Can you work these out from the model? Positions are in its coordinate system, mm. Face numbers are marked on the shaded views. A direction names the side the tool comes from. Round coordinates to 2 decimals unless told otherwise and drop trailing zeros. Order: outer loops, then holes, each group sorted by start corner. A loop starts at its lowest first (then second) coordinate and runs counter-clockwise, first axis right, second up. Notation, with made-up numbers: (14.5, 41.25) -> (44.5, 41.25) arc R25 cw to (44.5, 56.25) -> close; hole circle Ø6 at (55.25, 16). An arc over 180 degrees is marked (long way). Use a Markdown table: item, result. Add a question column.
Q1. If we section it at D-D on y = 15: List the corners of the cut face in (x, z) for me.
Q2. If we section it at A-A on z = -19.5: List the corners of the cut face in (x, y) for me.
Q3. For the marked faces 1, 2, 3, 4 and 5, which set-ups out of +Z, -Z, +X, -X, +Y, -Y let a thin tool reach every point of the face, with its end or its side?
Q4. I need wall thicknesses on line 1 along X through (y, z) = (-17, -2); line 2 along Z through (x, y) = (-14.5, -19). Which ranges of each line are inside material? Lowest first, please. Write a range as [from, to].
Q5. I'm going to push flat-ended pins straight in: pin 1 Ø1.5 at (x, y) = (-5, -7) entering from +Z; pin 2 Ø6 at (y, z) = (5, 5.5) entering from +X; pin 3 Ø6 at (y, z) = (-6, -14.5) entering from -X. Where does each tip first touch, or does it pass through?
Q6. We'd pull the mould along X, two halves only. Please class the marked faces 6, 7, 8 and 9: +X half, -X half, draft (parallel to the pull), parting line (faces both ways), or undercut.
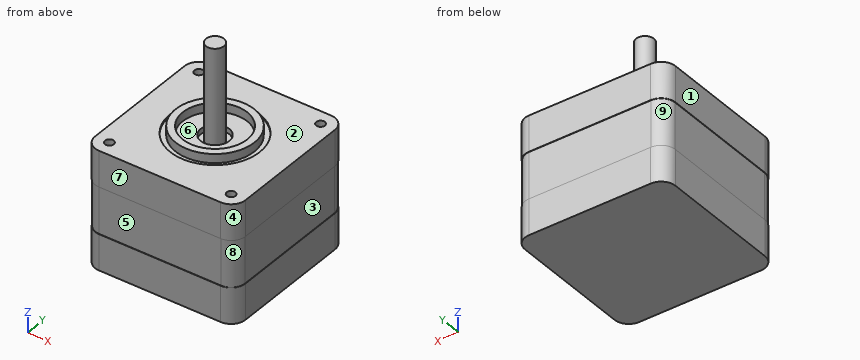
Autodesk Inventor part; units mm, degrees
ref_plane "Work Plane1" through (0, 0, -10) normal (0, 0, 1) x (1, 0, 0)
ref_plane "Work Plane3" through (0, 0, -23) normal (0, 0, 1) x (1, 0, 0)
ref_plane "YZ Plane" through (0, 0, 0) normal (1, 0, 0) x (0, 1, 0)
sketch "Sketch1" plane through (0, 0, 0) normal (0, 0, 1) x (1, 0, 0)
  circle A0 centre (0, 0) radius 12.5
  circle A1 centre (0, 0) radius 9
  circle A2 centre (0, 0) radius 11
  line L0 (17, -21) -> (-17, -21)
  line L1 (-21, -17) -> (-21, 17)
  line L2 (-17, 21) -> (17, 21)
  line L3 (21, 17) -> (21, -17)
  line L4 (21, -21) -> (-21, 21) construction
  line L5 (-21, -21) -> (21, 21) construction
  arc A3 (-17, 21) -> (-21, 17) centre (-17, 17) ccw
  arc A4 (-21, -17) -> (-17, -21) centre (-17, -17) ccw
  arc A5 (17, -21) -> (21, -17) centre (17, -17) ccw
  arc A6 (21, 17) -> (17, 21) centre (17, 17) ccw
  line L6 (15.5, -15.5) -> (-15.5, -15.5) construction
  line L7 (-15.5, -15.5) -> (-15.5, 15.5) construction
  line L8 (-15.5, 15.5) -> (15.5, 15.5) construction
  line L9 (15.5, 15.5) -> (15.5, -15.5) construction
  line L10 (15.5, -15.5) -> (-15.5, 15.5) construction
  line L11 (-15.5, -15.5) -> (15.5, 15.5) construction
  circle A7 centre (0, 0) radius 2.5
  circle A8 centre (0, 0) radius 4
  dimension "d0" = 42
  dimension "d2" = 42
  dimension "d3" = 4
  dimension "d4" = 18
  dimension "d5" = 22
  dimension "d6" = 25
  dimension "d7" = 31
  dimension "d22" = 5
  dimension "d23" = 8
ref_plane "Work Plane1" through (0, 0, -10) normal (0, 0, 1) x (1, 0, 0)
ref_plane "Work Plane3" through (0, 0, -23) normal (0, 0, 1) x (1, 0, 0)
ref_plane "Work Plane2" through (0, 0, -33) normal (0, 0, 1) x (1, 0, 0)
extrude "Extrusion1" add sketch "Sketch1" against normal up to surface (10 mm away) from surface at 0 contours A0 | A1 | A2 | L0 A4 L1 A3 L2 A6 L3 A5 | A7 | A8
sketch "Sketch2" plane through (17, 21, -10) normal (0, 0, -1) x (-1, 0, 0)
  arc A0 (34, -42) -> (38, -38) centre (34, -38) ccw
  line L0 (38, -38) -> (38, -4)
  arc A1 (38, -4) -> (34, 0) centre (34, -4) ccw
  line L1 (34, 0) -> (0, 0)
  arc A2 (0, 0) -> (-4, -4) centre (0, -4) ccw
  line L2 (-4, -4) -> (-4, -38)
  arc A3 (-4, -38) -> (0, -42) centre (0, -38) ccw
  line L3 (0, -42) -> (34, -42)
  line L4 (0, -0.1) -> (34, -0.1)
  arc A4 (37.9, -4) -> (34, -0.1) centre (34, -4) ccw
  line L5 (37.9, -4) -> (37.9, -38)
  arc A5 (34, -41.9) -> (37.9, -38) centre (34, -38) ccw
  line L6 (34, -41.9) -> (0, -41.9)
  arc A6 (-3.9, -38) -> (0, -41.9) centre (0, -38) ccw
  line L7 (-3.9, -38) -> (-3.9, -4)
  arc A7 (0, -0.1) -> (-3.9, -4) centre (0, -4) ccw
  point P0 (17, -21)
  dimension "d13" = 0.1
extrude "Extrusion2" add sketch "Sketch2" along normal up to surface (10 mm away) from surface at 13 contours L3 A3 L2 A2 L1 A1 L0 A0 | L4 A4 L5 A5 L6 A6 L7 A7
extrude "Extrusion3" add sketch "Sketch2" along normal up to surface (13 mm away) from surface at 0 contours L4 A4 L5 A5 L6 A6 L7 A7
extrude "Extrusion4" cut sketch "Sketch1" against normal blind 0.5 contours A0 | A1 | A8
extrude "Extrusion5" add sketch "Sketch1" along normal blind 2 contours A2
extrude "Extrusion6" cut sketch "Sketch1" against normal blind 2 contours A8
extrude "Extrusion7" add sketch "Sketch1" along normal blind 25 contours A7
hole "Hole1" at (-17, 17, 0) at (-17, -17, 0) at (17, -17, 0) at (17, 17, 0) direction (0, 0, -1) diameter 2.459 depth 4 tip angle 118
properties part number "nema17 33mm"
Answer below:
| question | item | result |
|---|---|---|
| 1 | outline | (-21, -33) -> (21, -33) -> (21, -23) -> (20.9, -23) -> (20.9, -10) -> (21, -10) -> (21, 0) -> (-21, 0) -> (-21, -10) -> (-20.9, -10) -> (-20.9, -23) -> (-21, -23) -> close |
| 2 | outline | (-20.9, -17) arc R3.9 ccw to (-17, -20.9) -> (17, -20.9) arc R3.9 ccw to (20.9, -17) -> (20.9, 17) arc R3.9 ccw to (17, 20.9) -> (-17, 20.9) arc R3.9 ccw to (-20.9, 17) -> close |
| 3 | face 1 | +Z, -Z, -X, +Y, -Y |
| 3 | face 2 | +Z |
| 3 | face 3 | +X, +Y, -Y |
| 3 | face 4 | +Z, -Z, +X, -Y |
| 3 | face 5 | +X, -X, -Y |
| 4 | line 1 | [-21, -18.23], [-15.77, 15.77], [18.23, 21] |
| 4 | line 2 | [-33, 0] |
| 5 | pin 1 | z = 2 |
| 5 | pin 2 | x = 1.5 |
| 5 | pin 3 | x = -20.9 |
| 6 | face 6 | undercut |
| 6 | face 7 | draft |
| 6 | face 8 | +X half |
| 6 | face 9 | -X half |
